Part print with two shaded views. Sizes in mm from the minimum x, y, z corner. A direction names the side the tool comes from. Give positions to 0.01 mm unless a question says otherwise; leave off trailing zeros. Order: outer loops, then holes, each group sorted by start corner. A loop starts at its lowest first (then second) coordinate and runs counter-clockwise, first axis right, second up. Notation, with made-up numbers: (65.5, 62.25) - (73.5, 62.25) arc R20 ccw to (73.5, 68.25) - close; hole circle Ø2 at (79, 19). An arc over 180 degrees is marked (long way). Return JSON: item names as keys, results as strings. Group by question number.
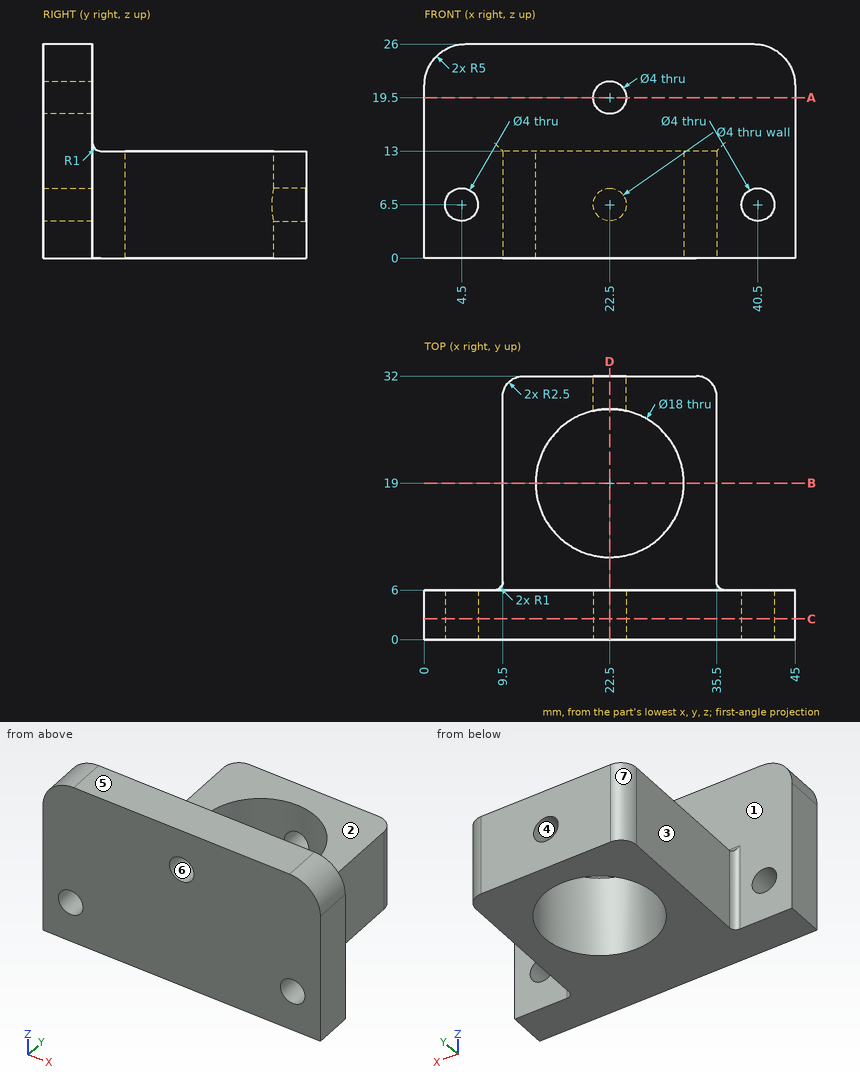
(1) Pull direction Z, two halves, no side cores. Call the marked faces 5, 6 and 7: released by +Z, released by -Z, zero draft, split by the parting line, or undercut.
(2) Drill centre lines: L1, parallel to X at y = 2.7, z = 6.5; L2, parallel to Z at x = 4, y = 1; L3, parallel to Y at x = 41, z = 16.5. Where is each one in solid material? Low to high.
(3) Slice it at A-A (z = 19.5). Give the cut face in (x, y).
(4) Drop flat-ended pins along their axis: pin 1 Ø4 at (y, z) = (28.5, 7.5) entering from -X; pin 2 Ø5 at (x, z) = (6.5, 21) entering from +Y; pin 3 Ø8 at (y, z) = (13.5, 12) entering from +X; pin 4 Ø3 at (x, z) = (22.5, 19.5) entering from -Y. Give the stop position or say it passes through.
(5) 3-axis set-ups, long thin cutter, end or side, ignore diameter. For the marked faces 1, 2, 3 and 4: which of +Z, -Z, +X, -X, +Y, -Y reach the whole face in a straight line?
(6) Slice it at B-B (y = 19). Give the cut face in (x, z), and give its area (3 significant figures).
(7) Slice it at D-D (x = 22.5). Give the cut face in (y, z), and give its area (3 significant figures).
(8) Slice it at C-C (y = 2.5). Give the cut face in (x, z).
Result set:
{
 "1": {"face 5": "released by +Z", "face 6": "undercut", "face 7": "zero draft"},
 "2": {"L1": "x = 0 to 2.5, 6.5 to 38.5, 42.5 to 45", "L2": "z = 0 to 4.56, 8.44 to 25.9", "L3": "y = 0 to 6"},
 "3": {"outline": "(0, 0) - (20.5, 0) - (20.5, 6) - (0, 6) - close; (24.5, 0) - (45, 0) - (45, 6) - (24.5, 6) - close"},
 "4": {"pin 1": "stops at x = 9.5", "pin 2": "stops at y = 6", "pin 3": "stops at x = 35.5", "pin 4": "passes through"},
 "5": {"face 1": "+Z, +Y", "face 2": "+Z, +X, -X, +Y", "face 3": "+Z, -Z, -X, +Y", "face 4": "+Y"},
 "6": {"outline": "(9.5, 0) - (13.5, 0) - (13.5, 13) - (9.5, 13) - close; (31.5, 0) - (35.5, 0) - (35.5, 13) - (31.5, 13) - close", "area": "104 mm²"},
 "7": {"outline": "(0, 0) - (10, 0) - (10, 13) - (7, 13) arc R1 cw to (6, 14) - (6, 17.5) - (0, 17.5) - close; (0, 21.5) - (6, 21.5) - (6, 26) - (0, 26) - close; (28, 0) - (32, 0) - (32, 4.5) - (28, 4.5) - close; (28, 8.5) - (32, 8.5) - (32, 13) - (28, 13) - close", "area": "220 mm²"},
 "8": {"outline": "(0, 0) - (45, 0) - (45, 21) arc R5 ccw to (40, 26) - (5, 26) arc R5 ccw to (0, 21) - close; hole circle Ø4 at (4.5, 6.5); hole circle Ø4 at (22.5, 19.5); hole circle Ø4 at (40.5, 6.5)"}
}
